Study the drawing (mm; zero at the part's minimum x, y, z) and answer. A direction names the side the tool comes from. Coordinates: 2 decimals unless noted, no trailing zeros. Order: outer loops, then holes, each group sorted by start corner. A loop starts at its lowest first (then second) coordinate and runs counter-clockwise, first axis right, second up.
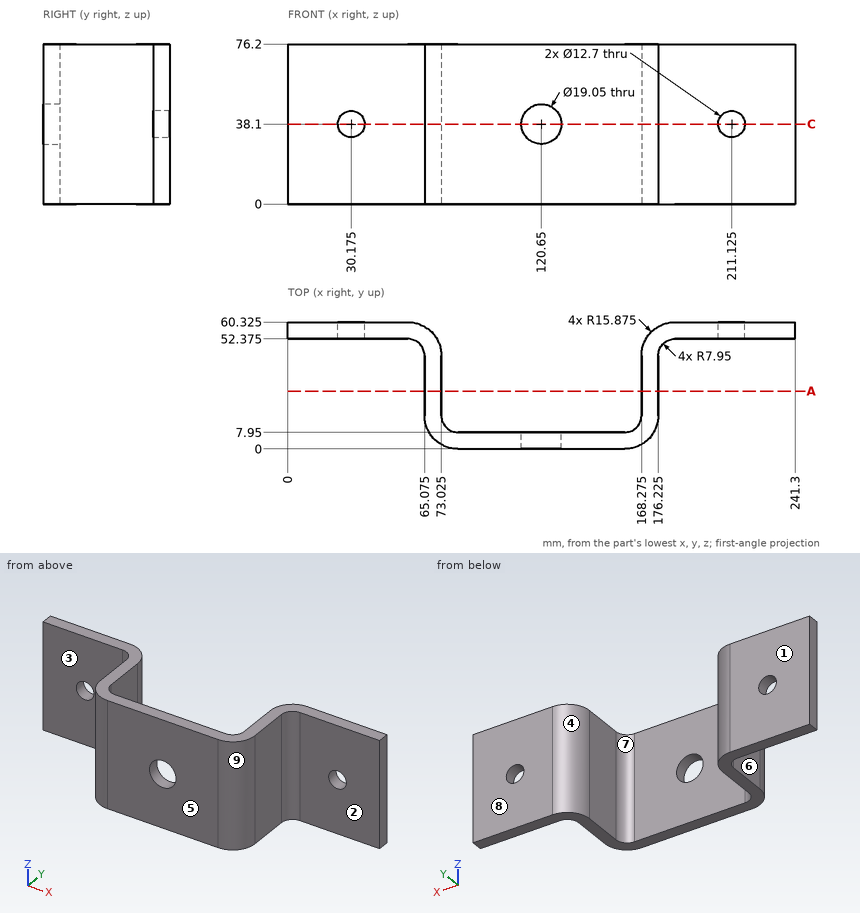
1) A cutting plane is placed at C-C, the plane z = 38.1. State how many separate pieces and enclosed holes the cut face has, and give its area (3 significant figures).
A:
separate pieces: 4
enclosed holes: 0
area: 2,240 mm2
2) Flat-ended cylindrical pins translate along their axes: pin 1 Ø2 at (x, z) = (56.5, 66.5) entering from -Y; pin 2 Ø4 at (y, z) = (22, 33.5) entering from -X (3 decimals); pin 3 Ø10 at (x, z) = (151, 67.5) entering from +Y; pin 4 Ø10 at (x, z) = (211.12, 38.1) entering from -Y. Find the tip coordinate at first contact, or state that the pin passes through.
A:
pin 1: stops at y = 52.37
pin 2: stops at x = 65.075
pin 3: stops at y = 7.95
pin 4: passes through
3) A cutting plane is placed at A-A, the plane y = 27.5. Determine the outline of the cut face in (x, z) (1 decimal).
A:
outline: (65.1, 0) - (73, 0) - (73, 76.2) - (65.1, 76.2) - close; (168.3, 0) - (176.2, 0) - (176.2, 76.2) - (168.3, 76.2) - close
4) Which of the six approach directions +Z, -Z, +X, -X, +Y, -Y give full straight-line access (tool end or side, diameter ignored) to the marked faces 1, 2, 3, 4 and 5?
A:
face 1: +Z, -Z, +X, -X, +Y
face 2: +Z, -Z, +X, -Y
face 3: +Z, -Z, -X, -Y
face 4: +Z, -Z, +Y
face 5: +Z, -Z, +X, -X, -Y
5) Straight lines are drawn through the part: line 1 (Z direction, x = 120, y = 2); line 2 (Y direction, x = 88, z = 24); line 3 (X direction, y = 53, z = 36) (1 decimal). For each, find the intervals that lie inside material, in ascending order.
A:
line 1: z = 0 to 28.6, 47.6 to 76.2
line 2: y = 0 to 7.95
line 3: x = 0 to 24.2, 36.2 to 70.5, 170.8 to 205.1, 217.1 to 241.3
6) Determine the mould class of the marked faces 6, 7, 8 and 9 for opening direction X: pulls with the +X half, pulls with the -X half, needs draft (parallel to the pull), parting line crosses it, or undercut.
A:
face 6: pulls with the -X half
face 7: undercut
face 8: needs draft
face 9: pulls with the +X half
